Could you check a few things on this model? Use its own coordinates, in mm. Round coordinates to 2 decimals unless told otherwise and drop trailing zeros. One line per question, with ' | ' between items. Start each with the question number.
1. For pin 1 Ø0.5 at (y, z) = (-14, 250.5) entering from +X; pin 2 Ø3 at (x, y) = (0, 9) entering from +Z; pin 3 Ø0.5 at (x, z) = (-14, 385.5) entering from -Y, each with a flat end and sliding along its axis, tell me the tip position at first contact or that it passes through.
2. If I drill on line 1 along X through (y, z) = (12.5, 70.5); line 2 along X through (y, z) = (-7.5, 584.5); line 3 along Y through (x, z) = (1.5, 531.5), over which ranges is the centre line in solid material (lowest first)? Write a range as [from, to].
3. Imagine slicing it at A-A, the plane z = 819. State how many separate pieces and enclosed holes the cut face has, and give its area (3 significant figures).
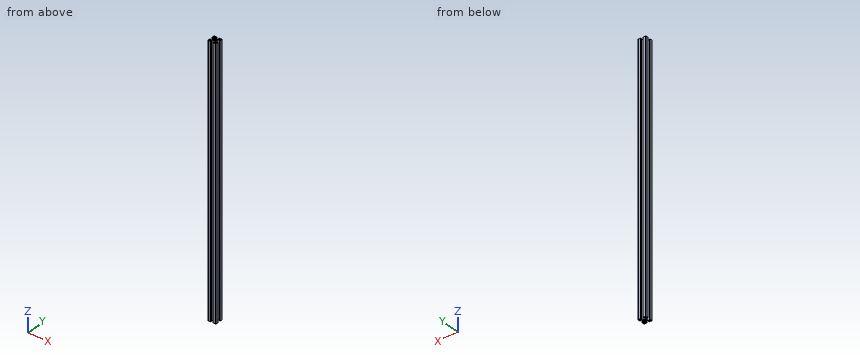
from build123d import *

# Parameters (mm, degrees)
F0_W     = 3
F0_H     = 3
F1_DEPTH = 1000
F2_R     = 1.5
F3_SIZE  = 0.6


with BuildPart() as f1:
    # F0 (on Top) → F1 (new body)
    with BuildSketch(Plane.XY):
        with BuildLine():
            Line((-4.1, 15), (-15, 15))
            Line((-15, 15), (-15, 4.1))
            Line((-15, 4.1), (-12.8, 4.1))
            Line((-12.8, 4.1), (-12.8, 9))
            Line((-12.8, 9), (-10.555635, 9))
            Line((-10.555635, 9), (-4.948549, 3.392914))
            ThreePointArc((-4.948549, 3.392914), (-6, 0), (-4.948549, -3.392914))
            Line((-4.948549, -3.392914), (-10.555635, -9))
            Line((-10.555635, -9), (-12.8, -9))
            Line((-12.8, -9), (-12.8, -4.1))
            Line((-12.8, -4.1), (-15, -4.1))
            Line((-15, -4.1), (-15, -15))
            Line((-15, -15), (-4.1, -15))
            Line((-4.1, -15), (-4.1, -12.8))
            Line((-4.1, -12.8), (-9, -12.8))
            Line((-9, -12.8), (-9, -10.555635))
            Line((-9, -10.555635), (-3.392914, -4.948549))
            ThreePointArc((-3.392914, -4.948549), (0, -6), (3.392914, -4.948549))
            Line((3.392914, -4.948549), (9, -10.555635))
            Line((9, -10.555635), (9, -12.8))
            Line((9, -12.8), (4.1, -12.8))
            Line((4.1, -12.8), (4.1, -15))
            Line((4.1, -15), (15, -15))
            Line((15, -15), (15, -4.1))
            Line((15, -4.1), (13.5, -4.1))
            Line((13.5, -4.1), (12.8, -4.1))
            Line((12.8, -4.1), (12.8, -9))
            Line((12.8, -9), (10.555635, -9))
            Line((10.555635, -9), (4.948549, -3.392914))
            ThreePointArc((4.948549, -3.392914), (6, 0), (4.948549, 3.392914))
            Line((4.948549, 3.392914), (10.555635, 9))
            Line((10.555635, 9), (12.8, 9))
            Line((12.8, 9), (12.8, 4.1))
            Line((12.8, 4.1), (13.5, 4.1))
            Line((13.5, 4.1), (15, 4.1))
            Line((15, 4.1), (15, 15))
            Line((15, 15), (4.1, 15))
            Line((4.1, 15), (4.1, 12.8))
            Line((4.1, 12.8), (9, 12.8))
            Line((9, 12.8), (9, 10.555635))
            Line((9, 10.555635), (3.392914, 4.948549))
            ThreePointArc((3.392914, 4.948549), (0, 6), (-3.392914, 4.948549))
            Line((-3.392914, 4.948549), (-9, 10.555635))
            Line((-9, 10.555635), (-9, 12.8))
            Line((-9, 12.8), (-4.1, 12.8))
            Line((-4.1, 12.8), (-4.1, 15))
        make_face()
        with Locations((-12, -12)):
            Rectangle(F0_W, F0_H, mode=Mode.SUBTRACT)
        with Locations((12, -12)):
            Rectangle(F0_W, F0_H, mode=Mode.SUBTRACT)
        with Locations((-12, 12)):
            Rectangle(F0_W, F0_H, mode=Mode.SUBTRACT)
        with BuildLine():
            ThreePointArc((2.94533, 1.890775), (3.358471, 0.985227), (3.5, 0))
            ThreePointArc((3.5, 0), (3.358471, -0.985227), (2.94533, -1.890775))
            ThreePointArc((2.94533, -1.890775), (3.223794, -2.434637), (3.005204, -3.005204))
            ThreePointArc((3.005204, -3.005204), (2.434637, -3.223794), (1.890775, -2.94533))
            ThreePointArc((1.890775, -2.94533), (0, -3.5), (-1.890775, -2.94533))
            ThreePointArc((-1.890775, -2.94533), (-2.434637, -3.223794), (-3.005204, -3.005204))
            ThreePointArc((-3.005204, -3.005204), (-3.223794, -2.434637), (-2.94533, -1.890775))
            ThreePointArc((-2.94533, -1.890775), (-3.5, 0), (-2.94533, 1.890775))
            ThreePointArc((-2.94533, 1.890775), (-3.223794, 2.434637), (-3.005204, 3.005204))
            ThreePointArc((-3.005204, 3.005204), (-2.434637, 3.223794), (-1.890775, 2.94533))
            ThreePointArc((-1.890775, 2.94533), (0, 3.5), (1.890775, 2.94533))
            ThreePointArc((1.890775, 2.94533), (2.434637, 3.223794), (3.005204, 3.005204))
            ThreePointArc((3.005204, 3.005204), (3.223794, 2.434637), (2.94533, 1.890775))
        make_face(mode=Mode.SUBTRACT)
        with Locations((12, 12)):
            Rectangle(F0_W, F0_H, mode=Mode.SUBTRACT)
    extrude(amount=F1_DEPTH)

    # F2
    f2_edges = [f1.edges().sort_by_distance(p)[0] for p in [
        (15, 15, 500),
        (-15, 15, 500),
        (15, -15, 500),
        (-15, -15, 500),
    ]]
    fillet(f2_edges, radius=F2_R)

    # F3
    f3_edges = [f1.edges().sort_by_distance(p)[0] for p in [
        (-4.1, 15, 500),
        (4.1, 15, 500),
        (15, 4.1, 500),
        (15, -4.1, 500),
        (-15, 4.1, 500),
        (-15, -4.1, 500),
        (4.1, -15, 500),
        (-4.1, -15, 500),
    ]]
    chamfer(f3_edges, length=F3_SIZE)


solid = f1.part
Geometry results:
1) pin 1: stops at x = 14.98 | pin 2: passes through | pin 3: stops at y = -14.98
2) line 1: x = [-15, -13.5], [-10.5, -9], [9, 10.5], [13.5, 15] | line 2: x = [-15, -12.8], [-9.06, -5.94], [5.94, 9.06], [12.8, 15] | line 3: y = [-5.81, -3.16], [3.16, 5.81]
3) separate pieces: 1 | enclosed holes: 5 | area: 326 mm2
